Answer from the drawing. Dimensions are ordinates in mm from the lowest x, y and z of the part. A direction names the side the tool comes from. Round coordinates to 2 decimals unless told otherwise and drop trailing zeros. Write each loop counter-clockwise with the first axis right and the second up, starting at its lowest first coordinate (ties: lowest second). Pieces come first, ordered by that corner, then holes.
1. Straight lines are drawn through the part: probe 1 along Z at (x, y) = (69.5, 47.1); probe 2 along Y at (x, z) = (118, 1.8); probe 3 along Z at (x, y) = (53, 37). For each, find the intervals that lie inside material, in ascending order.
2. A tool of negligible diameter and unlimited length cuts with its end or side. For the marked faces 4, 5, 6 and 7, from which of +Z, -Z, +X, -X, +Y, -Y can it reach the whole face along a straight path? Write none if from no direction.
3. Find section C-C (x = 118). Write down the section's boundary in (y, z).
4. Find section D-D (z = 62). Write down the section's boundary in (x, y).
5. Determine the mould class of the marked faces 1, 2 and 3 for opening direction X: pulls with the +X half, pulls with the -X half, needs draft (parallel to the pull), parting line crosses it, or undercut.
6. Find section B-B (x = 69.5). Write down the section's boundary in (y, z), and give its area (3 significant figures).
7. Find section A-A (y = 84). Write down the section's boundary in (x, z).
8. Flat-ended cylindrical pins translate along their axes: pin 1 Ø4 at (x, z) = (79.5, 26.5) entering from +Y; pin 2 Ø16 at (x, y) = (69.5, 21) entering from -Z; pin 3 Ø20.5 at (y, z) = (60.5, 30) entering from +X; pin 4 Ø22 at (x, y) = (21, 65) entering from +Z. Find the tip coordinate at first contact, or state that the pin passes through.
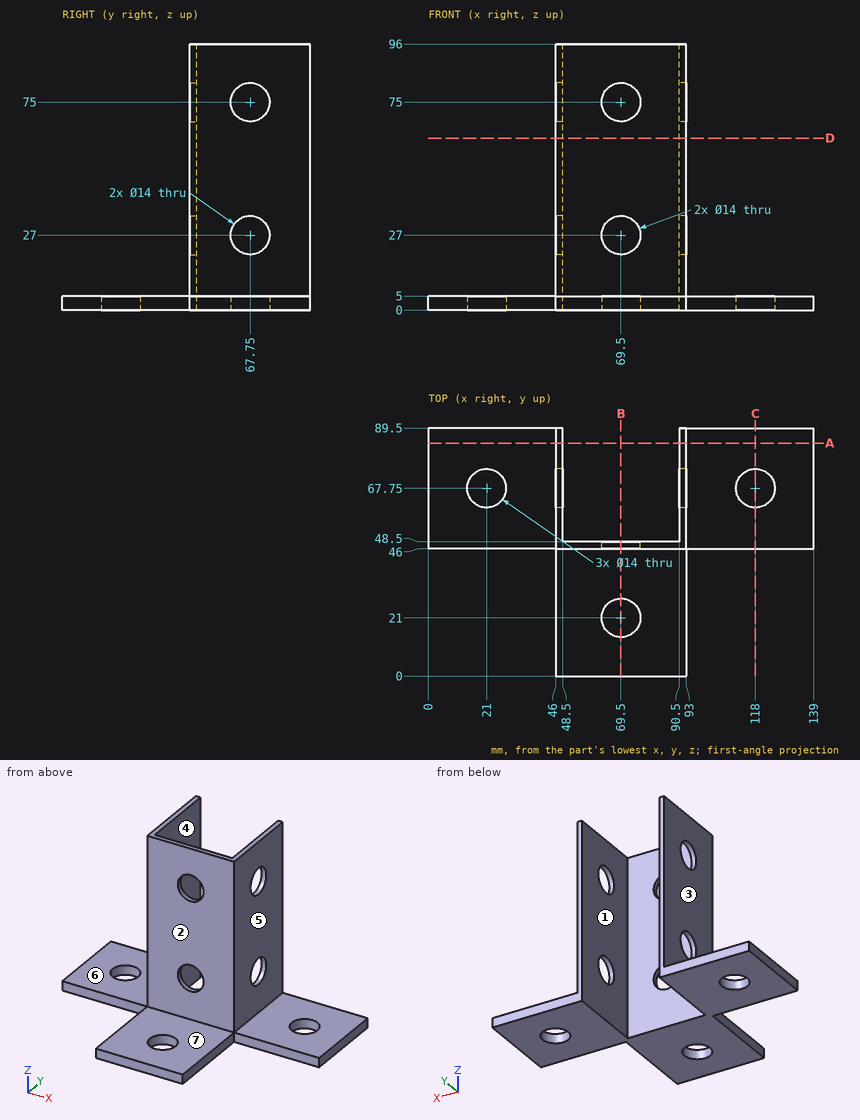
Worked answers:
1. probe 1: z = 0 to 20, 34 to 68, 82 to 96
1. probe 2: y = 46 to 60.75, 74.75 to 89.5
1. probe 3: z = 0 to 5
2. face 4: +Z, -Z, +Y
2. face 5: +Z, +X, +Y, -Y
2. face 6: +Z, -X, +Y, -Y
2. face 7: +Z, +X, -X, -Y
3. outline: (46, 0) - (60.75, 0) - (60.75, 5) - (46, 5) - close; (74.75, 0) - (89.5, 0) - (89.5, 5) - (74.75, 5) - close
4. outline: (46, 46) - (93, 46) - (93, 89.5) - (90.5, 89.5) - (90.5, 48.5) - (48.5, 48.5) - (48.5, 89.5) - (46, 89.5) - close
5. face 1: undercut
5. face 2: needs draft
5. face 3: pulls with the -X half
6. outline: (0, 0) - (14, 0) - (14, 5) - (0, 5) - close; (28, 0) - (48.5, 0) - (48.5, 20) - (46, 20) - (46, 5) - (28, 5) - close; (46, 34) - (48.5, 34) - (48.5, 68) - (46, 68) - close; (46, 82) - (48.5, 82) - (48.5, 96) - (46, 96) - close
6. area: 330 mm2
7. outline: (0, 0) - (48.5, 0) - (48.5, 96) - (46, 96) - (46, 5) - (0, 5) - close; (90.5, 0) - (139, 0) - (139, 5) - (93, 5) - (93, 96) - (90.5, 96) - close
8. pin 1: stops at y = 48.5
8. pin 2: stops at z = 0
8. pin 3: stops at x = 93
8. pin 4: stops at z = 5
